For this review, take the finished solid that the model builds, in its own axes (mm). A direction names the side the tool comes from. Coordinates: 2 decimals unless noted, no trailing zeros. Loops run counter-clockwise (first coordinate to the right, second up) from the corner with the lowest first, then second, coordinate; pieces in that order, holes last. Notation, with made-up numbers: (-7.5, 63.5) -> (26.5, 63.5) arc R27 ccw to (26.5, 97.5) -> close; hole circle Ø8 at (19, -33). An arc over 180 degrees is marked (long way). One line per item, written item: value.
from build123d import *

# Parameters (mm, degrees)
SKETCH1_W                 = 90
SKETCH1_H                 = 50
BOSS_EXTRUDE1_DEPTH       = 11.999999994
BOSS_EXTRUDE2_DEPTH       = 35
SKETCH3_W                 = 50
SKETCH3_H                 = 12
BOSS_EXTRUDE3_DEPTH       = 105
SKETCH4_W                 = 32.855882012
SKETCH4_H                 = 179.2
CUT_EXTRUDE1_DEPTH        = 32
CUT_EXTRUDE2_REACH        = 250.023
DRAFT1_ANGLE              = 5.699999999
M13_CLEARANCE_HOLE1_D     = 15.88
M13_CLEARANCE_HOLE2_D     = 15.88
M13_CLEARANCE_HOLE2_DEPTH = 140
M13_CLEARANCE_HOLE3_D     = 15.88
FILLET1_R                 = 3.5
FILLET2_R                 = 7


with BuildPart() as part:
    # Sketch1 → Boss-Extrude1 (new body)
    with BuildSketch(Plane.XZ.offset(-179.2)):
        with Locations((45, 0)):
            Rectangle(SKETCH1_W, SKETCH1_H)
    extrude(amount=-BOSS_EXTRUDE1_DEPTH)

    # Sketch2 → Boss-Extrude2 (add)
    with BuildSketch(Plane(origin=(0, 0, 0), x_dir=(0, -1, 0), z_dir=(-1, 0, 0))):
        Polygon((-0.5, -25), (0, -24.5), (0, -25), (12, -25), (12, 25), (0, 25), (0, 24.5), (-0.500000019, 25), (-178.7, 25), (-179.2, 24.5), (-179.2, -24.5), (-178.7, -25), align=None)
    extrude(amount=-BOSS_EXTRUDE2_DEPTH)

    # Sketch3 → Boss-Extrude3 (add)
    with BuildSketch(Plane(origin=(35, 0, 0), x_dir=(0, 0, -1), z_dir=(1, 0, 0))):
        with Locations((0, -5.999999989)):
            Rectangle(SKETCH3_W, SKETCH3_H)
    extrude(amount=BOSS_EXTRUDE3_DEPTH)

    # Sketch4 → Cut-Extrude1 (cut)
    with BuildSketch(Plane(origin=(35, 0, 0), x_dir=(0, 0, -1), z_dir=(1, 0, 0))):
        with Locations((0, 89.600000011)):
            Rectangle(SKETCH4_W, SKETCH4_H)
    extrude(amount=-CUT_EXTRUDE1_DEPTH, mode=Mode.SUBTRACT)

    # Sketch5 → Cut-Extrude2 (cut, up to next)
    with BuildSketch(Plane.XZ.offset(12), mode=Mode.PRIVATE) as cut_extrude2_sk1:
        with BuildLine():
            Line((125, 7.94), (20, 7.94))
            ThreePointArc((20, 7.94), (12.06, 0), (20, -7.94))
            Line((20, -7.94), (125, -7.94))
            ThreePointArc((125, -7.94), (132.94, 0), (125, 7.94))
        make_face()
    cut_extrude2_tool1 = extrude(cut_extrude2_sk1.sketch, amount=-CUT_EXTRUDE2_REACH, mode=Mode.PRIVATE) & part.part
    add(cut_extrude2_tool1.solids().sort_by_distance((72.5, -12, 0))[0], mode=Mode.SUBTRACT)

    # Draft1
    draft1_faces = [part.faces().sort_by_distance(p)[0] for p in [
        (19, 89.600000011, -16.427941006),
        (19, 89.600000011, 16.427941006),
    ]]
    draft(draft1_faces, Plane(origin=(3, 0, 0), x_dir=(0, 0, 1), z_dir=(1, 0, 0)), DRAFT1_ANGLE)

    # M13 Clearance Hole1 (through all)
    with Locations(Plane(origin=(3, 0, 0), x_dir=(0, 0, -1), z_dir=(1, 0, 0))):
        with Locations((0, 38.8)):
            Hole(M13_CLEARANCE_HOLE1_D / 2)

    # M13 Clearance Hole2
    with Locations(Plane.ZY):
        with Locations((0, 89.6), (0, 115), (0, 140.4), (0, 165.8)):
            Hole(M13_CLEARANCE_HOLE2_D / 2, depth=M13_CLEARANCE_HOLE2_DEPTH)

    # M13 Clearance Hole3 (through all)
    with Locations(Plane(origin=(0, 179.2, 0), x_dir=(-1, 0, 0), z_dir=(0, -1, 0))):
        with Locations((-76.2, 0), (-25.4, 0)):
            Hole(M13_CLEARANCE_HOLE3_D / 2)

    # Fillet1
    fillet1_edges = [part.edges().sort_by_distance(p)[0] for p in [
        (35, 89.6, 19.621965629),
        (35, 89.6, -19.621965629),
    ]]
    fillet(fillet1_edges, radius=FILLET1_R)

    # Fillet2
    fillet2_edges = [part.edges().sort_by_distance(p)[0] for p in [
        (3, 89.6, 16.427941006),
        (3, 89.6, -16.427941006),
    ]]
    fillet(fillet2_edges, radius=FILLET2_R)


solid = part.part
1. Insertion check: pin 1 Ø5 at (y, z) = (46, -17.5) entering from +X; pin 2 Ø2.5 at (y, z) = (128, -24.5) entering from +X; pin 3 Ø13 at (y, z) = (185.5, 10) entering from +X. Each pin has a flat end and moves straight along its axis. Give the tip position at first contact, or say it passes through.
Return value:
pin 1: stops at x = 33.61
pin 2: stops at x = 35
pin 3: stops at x = 90
2. Take a section at A-A, the plane x = 40. Give the boundary of the cut face in (y, z), and give its area (3 significant figures).
Return value:
outline: (-12, -25) -> (0, -25) -> (0, -7.94) -> (-12, -7.94) -> close; (-12, 7.94) -> (0, 7.94) -> (0, 25) -> (-12, 25) -> close; (179.2, -25) -> (191.2, -25) -> (191.2, 25) -> (179.2, 25) -> close
area: 1,010 mm2
3. Take a section at C-C, the plane y = 38.8. Give the boundary of the cut face in (x, z), and give its area (3 significant figures).
Return value:
outline: (0, -25) -> (35, -25) -> (35, -22.79) arc R3.5 ccw to (31.85, -19.31) -> (9.3, -17.06) arc R7 cw to (3, -10.09) -> (3, -7.94) -> (0, -7.94) -> close; (0, 7.94) -> (3, 7.94) -> (3, 10.09) arc R7 cw to (9.3, 17.06) -> (31.85, 19.31) arc R3.5 ccw to (35, 22.79) -> (35, 25) -> (0, 25) -> close
area: 561 mm2
4. Take a section at B-B, the plane x = 122.5. Give the boundary of the cut face in (y, z).
Return value:
outline: (-12, -25) -> (0, -25) -> (0, -7.94) -> (-12, -7.94) -> close; (-12, 7.94) -> (0, 7.94) -> (0, 25) -> (-12, 25) -> close
5. To check wall thickness, follow probe 1 along Y at (x, z) = (1, 0); probe 2 along Y at (x, z) = (50.5, 12); probe 3 along Z at (x, y) = (25, 184). State the ranges of each line that lie inside material, in increasing order. Write a range as from..to.
Return value:
probe 1: y = -12..30.86, 46.74..81.66, 97.54..107.06, 122.94..132.46, 148.34..157.86, 173.74..191.2
probe 2: y = -12..0, 179.2..191.2
probe 3: z = -25..-7.93, 7.93..25
6. For faces 1 (the flat face through (20.734, 88.346, -18.198)), 2 (the flat face through (73, -6, 7.94)), 3 (the flat face through (90, 185, 0)), list the 3-axis set-ups (+Z, -Z, +X, -X, +Y, -Y) from which the entire face can be reached by the end or side of a thin tool; tool diameter is ignored.
Return value:
face 1: +X
face 2: -Y
face 3: +Z, -Z, +X, +Y
7. Take a section at D-D, the plane x = 76.2. Give the boundary of the cut face in (y, z), and give its area (3 significant figures).
Return value:
outline: (-12, -25) -> (0, -25) -> (0, -7.94) -> (-12, -7.94) -> close; (-12, 7.94) -> (0, 7.94) -> (0, 25) -> (-12, 25) -> close; (179.2, -25) -> (191.2, -25) -> (191.2, -7.94) -> (179.2, -7.94) -> close; (179.2, 7.94) -> (191.2, 7.94) -> (191.2, 25) -> (179.2, 25) -> close
area: 819 mm2
8. The part is to be moulded in two halves that separate along X. For faces 4 (the cylindrical face through (4.859, 90.854, -14.843)), 5 (the flat face through (17, 88, 25)), 6 (the flat face through (72, -6, -7.94)), say which applies: pulls with the +X half, pulls with the -X half, needs draft (parallel to the pull), parting line crosses it, or undercut.
Return value:
face 4: pulls with the +X half
face 5: needs draft
face 6: undercut
